Autodesk Inventor part; units mm, degrees
ref_plane "dia1_XY" through (-6.35, 5.5499, 0) normal (1, 0, 0) x (0, 0, -1)
ref_plane "dia1_YZ" through (-6.35, 5.5499, 0) normal (0, 0, -1) x (0, 1, 0)
ref_plane "dia1_ZX" through (-6.35, 5.5499, 0) normal (0, 1, 0) x (1, 0, 0)
sketch "Sketch_1" plane through (0, 0, 0) normal (0, 0, 1) x (1, 0, 0)
  line L0 (636.6256, 0) -> (-6.35, 0)
  line L1 (-6.35, 0) -> (-6.35, 5.5499)
  line L2 (-6.35, 5.5499) -> (609.6, 5.5499)
  line L3 (609.6, 5.5499) -> (609.6, 15.9703)
  line L4 (609.6, 15.9703) -> (636.6256, 15.9703)
  line L5 (636.6256, 15.9703) -> (636.6256, 0)
  line L6 (636.6256, 0) -> (-6.35, 0)
revolve "Revolution1" add sketch "Sketch_1" angle 360 about axis through (636.6256, 0, 0) along (1, 0, 0)
sketch "Sketch_3" plane through (0, 0, 0) normal (0, 0, 1) x (1, 0, 0)
  line L0 (-6.35, 0) -> (-25.4, 0)
  line L1 (-25.4, 0) -> (-25.4, 4.8006)
  line L2 (-25.4, 4.8006) -> (-24.6443, 5.5563)
  line L3 (-24.6443, 5.5563) -> (-6.35, 5.5563)
  line L4 (-6.35, 5.5563) -> (-6.35, 0)
  line L5 (-6.35, 0) -> (-25.4, 0)
revolve "Revolution2" add sketch "Sketch_3" angle 360 about axis through (-6.35, 0, 0) along (1, 0, 0)
thread "Thread1"
sketch "Sketch_10" plane through (-6.35, 0, 0) normal (1, 0, 0) x (0, 0, -1)
  line L0 (-11.0998, -11.0998) -> (11.0998, -11.0998)
  line L1 (11.0998, -11.0998) -> (11.0998, 11.0998)
  line L2 (11.0998, 11.0998) -> (-11.0998, 11.0998)
  line L3 (-11.0998, 11.0998) -> (-11.0998, -11.0998)
  line L4 (-4.826, -5.5499) -> (4.826, -5.5499)
  line L5 (4.826, -5.5499) -> (4.826, 5.5499)
  line L6 (4.826, 5.5499) -> (-4.826, 5.5499)
  line L7 (-4.826, 5.5499) -> (-4.826, -5.5499)
extrude "Extrusion1" cut sketch "Sketch_10" along normal blind 6.35
ref_plane "dia1_XY" through (-6.35, 5.5499, 0) normal (1, 0, 0) x (0, 0, -1)
ref_plane "dia1_YZ" through (-6.35, 5.5499, 0) normal (0, 0, -1) x (0, 1, 0)
ref_plane "dia1_ZX" through (-6.35, 5.5499, 0) normal (0, 1, 0) x (1, 0, 0)
ref_plane "dia12_XY" through (0, 0, 16.8466) normal (1, 0, 0) x (0, 0, -1)
ref_plane "dia12_YZ" through (0, 0, 16.8466) normal (0, 0, -1) x (0, 1, 0)
ref_plane "dia12_ZX" through (0, 0, 16.8466) normal (0, 1, 0) x (1, 0, 0)
ref_plane "dia2_XY" through (-6.35, -5.5499, 0) normal (1, 0, 0) x (0, 0, -1)
ref_plane "dia2_YZ" through (-6.35, -5.5499, 0) normal (0, 0, -1) x (0, 1, 0)
ref_plane "dia2_ZX" through (-6.35, -5.5499, 0) normal (0, 1, 0) x (1, 0, 0)
ref_plane "dia22_XY" through (0, 0, -16.8466) normal (1, 0, 0) x (0, 0, -1)
ref_plane "dia22_YZ" through (0, 0, -16.8466) normal (0, 0, -1) x (0, 1, 0)
ref_plane "dia22_ZX" through (0, 0, -16.8466) normal (0, 1, 0) x (1, 0, 0)
ref_plane "hh1_XY" through (669.1313, 0, 0) normal (0, 0, 1) x (1, 0, 0)
ref_plane "hh1_YZ" through (669.1313, 0, 0) normal (1, 0, 0) x (0, 1, 0)
ref_plane "hh1_ZX" through (669.1313, 0, 0) normal (0, 1, 0) x (0, 0, 1)
ref_plane "hh2_XY" through (675.5448, 0, 0) normal (0, 0, 1) x (1, 0, 0)
ref_plane "hh2_YZ" through (675.5448, 0, 0) normal (1, 0, 0) x (0, 1, 0)
ref_plane "hh2_ZX" through (675.5448, 0, 0) normal (0, 1, 0) x (0, 0, 1)
ref_plane "rl1_XY" through (-25.4, 0, 0) normal (1, 0, 0) x (0, 0, -1)
ref_plane "rl1_YZ" through (-25.4, 0, 0) normal (0, 0, -1) x (0, 1, 0)
ref_plane "rl1_ZX" through (-25.4, 0, 0) normal (0, 1, 0) x (1, 0, 0)
ref_plane "rl2_XY" through (-6.35, 0, 0) normal (1, 0, 0) x (0, 0, -1)
ref_plane "rl2_YZ" through (-6.35, 0, 0) normal (0, 0, -1) x (0, 1, 0)
ref_plane "rl2_ZX" through (-6.35, 0, 0) normal (0, 1, 0) x (1, 0, 0)
ref_plane "rod_cp_XY" through (0, 0, 0) normal (1, 0, 0) x (0, 0, -1)
ref_plane "rod_cp_YZ" through (0, 0, 0) normal (0, 0, -1) x (0, 1, 0)
ref_plane "rod_cp_ZX" through (0, 0, 0) normal (0, 1, 0) x (1, 0, 0)
ref_plane "thd1_XY" through (-25.4, 5.5563, 0) normal (1, 0, 0) x (0, 0, -1)
ref_plane "thd1_YZ" through (-25.4, 5.5563, 0) normal (0, 0, -1) x (0, 1, 0)
ref_plane "thd1_ZX" through (-25.4, 5.5563, 0) normal (0, 1, 0) x (1, 0, 0)
ref_plane "thd2_XY" through (-25.4, -5.5563, 0) normal (1, 0, 0) x (0, 0, -1)
ref_plane "thd2_YZ" through (-25.4, -5.5563, 0) normal (0, 0, -1) x (0, 1, 0)
ref_plane "thd2_ZX" through (-25.4, -5.5563, 0) normal (0, 1, 0) x (1, 0, 0)
ref_plane "to_rod_clevis_XY" through (-31.75, 0, 0) normal (1, 0, 0) x (0, 0, -1)
ref_plane "to_rod_clevis_YZ" through (-31.75, 0, 0) normal (0, 0, -1) x (0, 1, 0)
ref_plane "to_rod_clevis_ZX" through (-31.75, 0, 0) normal (0, 1, 0) x (1, 0, 0)
ref_plane "wf1_XY" through (-6.35, 0, 0) normal (1, 0, 0) x (0, 0, -1)
ref_plane "wf1_YZ" through (-6.35, 0, 0) normal (0, 0, -1) x (0, 1, 0)
ref_plane "wf1_ZX" through (-6.35, 0, 0) normal (0, 1, 0) x (1, 0, 0)
ref_plane "wf2_XY" through (0, 0, 0) normal (1, 0, 0) x (0, 0, -1)
ref_plane "wf2_YZ" through (0, 0, 0) normal (0, 0, -1) x (0, 1, 0)
ref_plane "wf2_ZX" through (0, 0, 0) normal (0, 1, 0) x (1, 0, 0)
ref_plane "wfw1_XY" through (-6.35, 0, -4.826) normal (0, 1, 0) x (1, 0, 0)
ref_plane "wfw1_YZ" through (-6.35, 0, -4.826) normal (1, 0, 0) x (0, 0, -1)
ref_plane "wfw1_ZX" through (-6.35, 0, -4.826) normal (0, 0, -1) x (0, 1, 0)
ref_plane "wfw2_XY" through (-6.35, 0, 4.826) normal (0, 1, 0) x (1, 0, 0)
ref_plane "wfw2_YZ" through (-6.35, 0, 4.826) normal (1, 0, 0) x (0, 0, -1)
ref_plane "wfw2_ZX" through (-6.35, 0, 4.826) normal (0, 0, -1) x (0, 1, 0)
properties part number "SR-1222-DP0000_rod"
Could you check a few things on this model? Use its own coordinates, in mm. A direction names the side the tool comes from. Give positions to 0.01 mm unless a question says otherwise; leave off trailing zeros. Loops run counter-clockwise (first coordinate to the right, second up) from the corner with the lowest first, then second, coordinate; pieces in that order, holes last. Notation, with made-up numbers: (27.25, 17) -> (34.25, 17) arc R27 ccw to (34.25, 53) -> close; hole circle Ø1 at (53, 43.5). An arc over 180 degrees is marked (long way). Answer as CSV lines item,"result". Start each with the question number.
(1) I'm going to push flat-ended pins straight in: pin 1 Ø0.8 at (y, z) = (-0.5, -5.5) entering from -X; pin 2 Ø3 at (x, z) = (552, 4) entering from +Y; pin 3 Ø4 at (x, z) = (280.5, -3.5) entering from -Y. Where does each tip first touch, or does it pass through?
(2) Which directions (+Z, -Z, +X, -X, +Y, -Y) give clear straight access to the entire face, cutting with the end or side of a thin tool? Please do faces 1 (the flat face through (636.626, 0, 0)), 2 (the cylindrical face through (305.937, 5.127, -2.126)).
(3) I need wall thicknesses on probe 1 along X at (y, z) = (-1.5, -13); probe 2 along Y at (x, z) = (589.5, 2.5); probe 3 along Y at (x, z) = (405.5, -3). Which ranges of each line are inside material? Lowest first, please.
(4) If we section it at B-B on x = 230: Write out the boundary of the cut face in (y, z), then the cut area to 3 significant figures.
Computed:
1,pin 1,"stops at x = -25.08"
1,pin 2,"stops at y = 4.95"
1,pin 3,"stops at y = -5.34"
2,face 1,"+Z, -Z, +X, +Y, -Y"
2,face 2,"-X"
3,probe 1,"x = 609.6 to 636.63"
3,probe 2,"y = -4.95 to 4.95"
3,probe 3,"y = -4.67 to 4.67"
4,outline,"circle Ø11.1 at (0, 0)"
4,area,"96.8 mm2"
